Read the model definition and answer for the solid it produces. Units are mm, in the model's axes. Face numbers are marked on the shaded views. A direction names the side the tool comes from. Give positions to 0.01 mm unless a question says otherwise; leave off trailing zeros. Loops run counter-clockwise (first coordinate to the right, second up) from the corner with the lowest first, then second, coordinate; pieces in that order, holes last. Notation, with made-up numbers: (21.5, -0.75) -> (75.5, -0.75) arc R9 cw to (75.5, 5.25) -> close; hole circle Ø9 at (44.5, -26.5). An arc over 180 degrees is marked (long way). One line per item, written item: value. Start each with the question number.
from build123d import *

# Parameters (mm, degrees)
SKETCH1_W           = 43.5
SKETCH1_H           = 17.8
SKETCH1_R           = 0.75
BOSS_EXTRUDE1_DEPTH = 1.8
SKETCH2_W           = 9.8
SKETCH2_H           = 7.8
BOSS_EXTRUDE2_DEPTH = 3.5
CUT_EXTRUDE1_DEPTH  = 46.5
SKETCH4_W           = 1.61922946
SKETCH4_H           = 3.886150706
CUT_EXTRUDE2_DEPTH  = 8.5
SKETCH5_W           = 38
SKETCH5_H           = 2.5
BOSS_EXTRUDE3_DEPTH = 3.2


with BuildPart() as part:
    # Sketch1 → Boss-Extrude1 (new body)
    with BuildSketch(Plane.XY):
        Rectangle(SKETCH1_W, SKETCH1_H)
        with Locations((20.75, 7.9)):
            Circle(SKETCH1_R, mode=Mode.SUBTRACT)
        with Locations((-20.75, 7.9)):
            Circle(SKETCH1_R, mode=Mode.SUBTRACT)
        with Locations((20.75, -7.9)):
            Circle(SKETCH1_R, mode=Mode.SUBTRACT)
        with Locations((-20.75, -7.9)):
            Circle(SKETCH1_R, mode=Mode.SUBTRACT)
    extrude(amount=BOSS_EXTRUDE1_DEPTH)

    # Sketch2 → Boss-Extrude2 (add)
    with BuildSketch(Plane.XY.offset(1.8)):
        with Locations((18.85, 0)):
            Rectangle(SKETCH2_W, SKETCH2_H)
    extrude(amount=BOSS_EXTRUDE2_DEPTH)

    # Sketch3 → Cut-Extrude1 (cut, through all)
    with BuildSketch(Plane(origin=(23.75, 0, 0), x_dir=(0, 0, -1), z_dir=(1, 0, 0))):
        with BuildLine():
            Line((-3.55, 3.9), (-1.8, 3.9))
            Line((-1.8, 3.9), (-1.8, 3.25))
            add(Edge.make_bspline(
                [(-1.8, 3.25), (-3.138543339, 3.528152874), (-3.55, 3.9)],
                knots=[0, 0, 0, 0.396074417, 0.396074417, 0.396074417], degree=2))
        make_face()
        with BuildLine():
            Line((-3.55, -3.9), (-1.8, -3.9))
            Line((-1.8, -3.9), (-1.8, -3.25))
            add(Edge.make_bspline(
                [(-1.8, -3.25), (-3.138543339, -3.528152874), (-3.55, -3.9)],
                knots=[0, 0, 0, 0.396074417, 0.396074417, 0.396074417], degree=2))
        make_face()
    extrude(amount=-CUT_EXTRUDE1_DEPTH, mode=Mode.SUBTRACT)

    # Sketch4 → Cut-Extrude2 (cut)
    with BuildSketch(Plane(origin=(23.75, 0, 0), x_dir=(0, 0, -1), z_dir=(1, 0, 0))):
        with BuildLine():
            Line((-3.55, -3.6), (-5.05, -3.6))
            Line((-5.05, -3.6), (-5.05, 3.6))
            Line((-5.05, 3.6), (-3.55, 3.6))
            add(Edge.make_bspline(
                [(-3.55, 3.6), (-2.837497732, 3.119257632), (-2.05, 3.105849487)],
                knots=[0, 0, 0, 0.945732544, 0.945732544, 0.945732544], degree=2))
            Line((-2.05, 3.105849487), (-2.05, -3.105849487))
            add(Edge.make_bspline(
                [(-3.55, -3.6), (-2.837497732, -3.119257632), (-2.05, -3.105849487)],
                knots=[0, 0, 0, 0.945732544, 0.945732544, 0.945732544], degree=2))
        make_face()
        with Locations((-3.55, 0)):
            Rectangle(SKETCH4_W, SKETCH4_H, mode=Mode.SUBTRACT)
    extrude(amount=-CUT_EXTRUDE2_DEPTH, mode=Mode.SUBTRACT)

    # Sketch5 → Boss-Extrude3 (add)
    with BuildSketch(Plane(origin=(0, 0, 0), x_dir=(-1, 0, 0), z_dir=(0, 0, -1))):
        with Locations((0, 7.65)):
            Rectangle(SKETCH5_W, SKETCH5_H)
        with Locations((0, -7.65)):
            Rectangle(SKETCH5_W, SKETCH5_H)
    extrude(amount=BOSS_EXTRUDE3_DEPTH)


solid = part.part
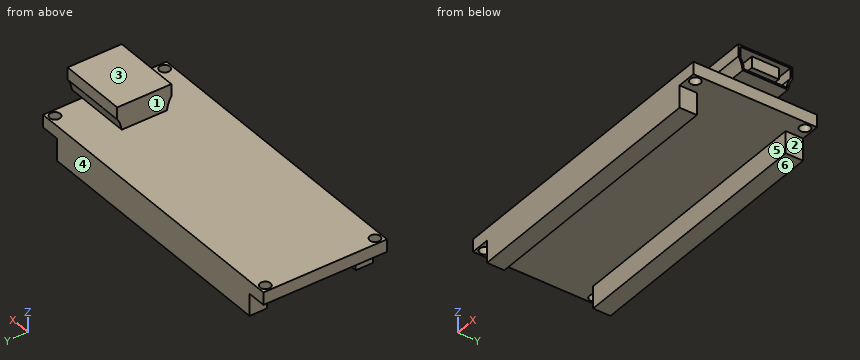
Item 1: Flat-ended cylindrical pins translate along their axes: pin 1 (1 mm diameter, centred on y = -3.5, z = 4.5, fed in from -X); pin 2 (2 mm diameter, centred on y = 7.5, z = -1.5, fed in from +X); pin 3 (0.8 mm diameter, centred on y = 8, z = -2.5, fed in from -X); pin 4 (1.2 mm diameter, centred on x = 20.75, y = -7.9, fed in from -Z). Find the tip coordinate at first contact, or state that the pin passes through.
Item 2: For the marked faces 1, 2 and 3, determine the directions among +Z, -Z, +X, -X, +Y, -Y from which every point of the face is accessible in a straight line to the end or side of a thin tool.
Item 3: Consider L1, parallel to Y at x = -20.75, z = 0.65; L2, parallel to Y at x = 17, z = -2.25; L3, parallel to X at y = -6.5, z = -2. Determine where each line is inside the solid, lowest interval first. Write a range as [from, to].
Item 4: Determine the mould class of the marked faces 4, 5 and 6 for opening direction Y: pulls with the +Y half, pulls with the -Y half, needs draft (parallel to the pull), parting line crosses it, or undercut.
Item 5: Section A-A, the plane z = -2 is taken. Determine the outline of the cut face in (x, y), plus the area to 3 significant figures.
Item 6: Section C-C, the plane x = 20.75 is taken. State how many separate pieces and enclosed holes the cut face has, plus the area to 3 significant figures.
Item 7: Section B-B, the plane y = -7.9 is taken. Determine the outline of the cut face in (x, z), plus the area to 4 significant figures.
Item 8: Section D-D, the plane z = 0.75 is taken. Determine the outline of the cut face in (x, y).
Computed values:
1. pin 1: x = 13.95
1. pin 2: x = 19
1. pin 3: x = -19
1. pin 4: through
2. face 1: +Z, -X, +Y, -Y
2. face 2: -Z, +X, +Y, -Y
2. face 3: +Z, +X, -X, +Y, -Y
3. L1: [-8.9, -8.65], [-7.15, 7.15], [8.65, 8.9]
3. L2: [-8.9, -6.4], [6.4, 8.9]
3. L3: [-19, 19]
4. face 4: pulls with the +Y half
4. face 5: undercut
4. face 6: needs draft
5. outline: (-19, -8.9) -> (19, -8.9) -> (19, -6.4) -> (-19, -6.4) -> close; (-19, 6.4) -> (19, 6.4) -> (19, 8.9) -> (-19, 8.9) -> close
5. area: 190 mm²
6. separate pieces: 4
6. enclosed holes: 1
6. area: 38.2 mm²
7. outline: (-21.75, 0) -> (-21.5, 0) -> (-21.5, 1.8) -> (-21.75, 1.8) -> close; (-20, 0) -> (-19, 0) -> (-19, -3.2) -> (19, -3.2) -> (19, 0) -> (20, 0) -> (20, 1.8) -> (-20, 1.8) -> close; (21.5, 0) -> (21.75, 0) -> (21.75, 1.8) -> (21.5, 1.8) -> close
7. area: 194.5 mm²
8. outline: (-21.75, -8.9) -> (21.75, -8.9) -> (21.75, 8.9) -> (-21.75, 8.9) -> close; hole circle Ø1.5 at (-20.75, -7.9); hole circle Ø1.5 at (-20.75, 7.9); hole circle Ø1.5 at (20.75, -7.9); hole circle Ø1.5 at (20.75, 7.9)
